Check sheet for the modelled part. Datum: model origin and axes. Units: mm. A direction names the side the tool comes from. Coordinates: 2 decimals unless noted, no trailing zeros. Order: outer loops, then holes, each group sorted by start corner. A loop starts at its lowest first (then second) coordinate and runs counter-clockwise, first axis right, second up.
1. Cross-section at C-C (y = -163.5). Enter the section's corners in (x, z), then the cut area to 3 significant figures.
2. Cross-section at D-D (y = -271). Enter the section's corners in (x, z).
3. Set-up check for faces 1 (the flat face through (2, -335, -29)), 2 (the flat face through (0, -165, 28)): record each of +Z, -Z, +X, -X, +Y, -Y from which the full face is reachable in a straight line by a thin tool's end or side.
4. Draft check along X on faces 3 (the flat face through (30, -165, 20)), 4 (the flat face through (28, -165, -19)), 5 (the flat face through (0, -165, -30)). Enter one of: released by +X, released by -X, zero draft, split by the parting line, or undercut.
5. Cross-section at B-B (x = 9). Enter the section's corners in (y, z), then the cut area to 3 significant figures.
6. Thickness scan on line 1 (Z direction, x = -20.5, y = -242.5). Record the ranges inside material, lowest first.
7. Cross-section at A-A (z = 9). Count the separate pieces of the cut face and the enclosed holes in it, then the cut area to 3 significant figures.
Autodesk Inventor part; units mm, degrees
ref_plane "YZ Plane" through (0, 0, 0) normal (1, 0, 0) x (0, 1, 0)
ref_plane "XZ Plane" through (0, 0, 0) normal (0, 1, 0) x (-1, 0, 0)
ref_plane "XY Plane" through (0, 0, 0) normal (0, 0, 1) x (1, 0, 0)
sketch "Sketch9" plane through (0, 0, 0) normal (0, 1, 0) x (-1, 0, 0)
  line L0 (30, 30) -> (-30, 30)
  line L1 (-30, 30) -> (-30, -30)
  line L2 (-30, -30) -> (30, -30)
  line L3 (30, -30) -> (30, 30)
  line L4 (30, 30) -> (-30, -30) construction
  line L5 (-30, 30) -> (30, -30) construction
  line L6 (-28, 28) -> (28, 28)
  line L7 (28, 28) -> (28, -28)
  line L8 (28, -28) -> (-28, -28)
  line L9 (-28, -28) -> (-28, 28)
  point P0 (0, 0)
  dimension "d172" = 60
  dimension "d173" = 60
  dimension "d174" = 2
extrude "Extrusion3" add sketch "Sketch9" against normal blind 335
sketch "Sketch10" plane through (0, 0, 0) normal (1, 0, 0) x (0, 1, 0)
  line L0 (0, 30) -> (0, -30) construction
  line L1 (0, 30) -> (-335, 30) construction
  line L2 (-335, -30) -> (-335, 30) construction
  line L3 (0, -30) -> (-335, -30) construction
  line L4 (-58.25, 15.25) -> (-27.75, 15.25)
  line L5 (-27.75, 15.25) -> (-27.75, -15.25)
  line L6 (-27.75, -15.25) -> (-58.25, -15.25)
  line L7 (-58.25, -15.25) -> (-58.25, 15.25)
  line L8 (-58.25, 15.25) -> (-27.75, -15.25) construction
  line L9 (-27.75, 15.25) -> (-58.25, -15.25) construction
  line L10 (-178.25, 15.25) -> (-147.75, 15.25)
  line L11 (-147.75, 15.25) -> (-147.75, -15.25)
  line L12 (-147.75, -15.25) -> (-178.25, -15.25)
  line L13 (-178.25, -15.25) -> (-178.25, 15.25)
  line L14 (-178.25, 15.25) -> (-147.75, -15.25) construction
  line L15 (-147.75, 15.25) -> (-178.25, -15.25) construction
  line L16 (-308.25, 15.25) -> (-277.75, 15.25)
  line L17 (-277.75, 15.25) -> (-277.75, -15.25)
  line L18 (-277.75, -15.25) -> (-308.25, -15.25)
  line L19 (-308.25, -15.25) -> (-308.25, 15.25)
  line L20 (-308.25, 15.25) -> (-277.75, -15.25) construction
  line L21 (-277.75, 15.25) -> (-308.25, -15.25) construction
  circle A0 centre (-453, 0) radius 9
  line L22 (0, 0) -> (47, 0)
  point P0 (-43, 0)
  point P1 (-163, 0)
  point P2 (-293, 0)
  dimension "d177" = 30.5
  dimension "d178" = 30.5
  dimension "d181" = 47
  dimension "d182" = 90
  dimension "d183" = 210
  dimension "d184" = 340
  dimension "d185" = 500
  dimension "d186" = 18
extrude "Extrusion4" cut sketch "Sketch10" along normal through all both and the other way through all contours L4 L5 L6 L7 | L10 L11 L12 L13 | L16 L17 L18 L19
sketch "Sketch11" plane through (30, 0, 30) normal (1, 0, 0) x (0, 0, -1)
  line L0 (45.25, -178.25) -> (14.75, -178.25)
  line L1 (14.75, -178.25) -> (14.75, -147.75)
  line L2 (14.75, -147.75) -> (45.25, -147.75)
  line L3 (45.25, -147.75) -> (45.25, -178.25)
  line L4 (45.25, -58.25) -> (14.75, -58.25)
  line L5 (14.75, -58.25) -> (14.75, -27.75)
  line L6 (14.75, -27.75) -> (45.25, -27.75)
  line L7 (45.25, -27.75) -> (45.25, -58.25)
  line L8 (45.25, -308.25) -> (14.75, -308.25)
  line L9 (14.75, -308.25) -> (14.75, -277.75)
  line L10 (14.75, -277.75) -> (45.25, -277.75)
  line L11 (45.25, -277.75) -> (45.25, -308.25)
  line L12 (0, 0) -> (60, 0)
  line L13 (0, 0) -> (0, -335)
  line L14 (60, -335) -> (0, -335)
  line L15 (60, 0) -> (60, -335)
  line L16 (45.25, -27.75) -> (14.75, -58.25)
  line L17 (45.25, -147.75) -> (14.75, -178.25)
  line L18 (45.25, -277.75) -> (14.75, -308.25)
  point P0 (30, 0)
sketch "Sketch13" plane through (-30, 0, -30) normal (-1, 0, 0) x (0, 0, 1)
  line L0 (45.25, -178.25) -> (14.75, -178.25)
  line L1 (14.75, -178.25) -> (14.75, -147.75)
  line L2 (14.75, -147.75) -> (45.25, -147.75)
  line L3 (45.25, -147.75) -> (45.25, -178.25)
  line L4 (45.25, -58.25) -> (14.75, -58.25)
  line L5 (14.75, -58.25) -> (14.75, -27.75)
  line L6 (14.75, -27.75) -> (45.25, -27.75)
  line L7 (45.25, -27.75) -> (45.25, -58.25)
  line L8 (45.25, -308.25) -> (14.75, -308.25)
  line L9 (14.75, -308.25) -> (14.75, -277.75)
  line L10 (14.75, -277.75) -> (45.25, -277.75)
  line L11 (45.25, -277.75) -> (45.25, -308.25)
  line L12 (0, 0) -> (60, 0)
  line L13 (0, 0) -> (0, -335)
  line L14 (60, -335) -> (0, -335)
  line L15 (60, 0) -> (60, -335)
  line L16 (14.75, -58.25) -> (45.25, -27.75)
  line L17 (14.75, -178.25) -> (45.25, -147.75)
  line L18 (14.75, -308.25) -> (45.25, -277.75)
  point P0 (30, 0)
fillet "Fillet1" radius 2 24 edges at (29, -277.75, -15.25) (29, -277.75, 15.25) (29, -308.25, 15.25) (29, -308.25, -15.25) (29, -178.25, -15.25) (29, -178.25, 15.25) (29, -147.75, 15.25) (29, -147.75, -15.25) (29, -58.25, 15.25) (29, -27.75, 15.25) (29, -27.75, -15.25) (29, -58.25, -15.25) (-29, -58.25, 15.25) (-29, -27.75, 15.25) (-29, -27.75, -15.25) (-29, -58.25, -15.25) (-29, -147.75, 15.25) (-29, -178.25, 15.25) (-29, -178.25, -15.25) (-29, -147.75, -15.25) (-29, -277.75, 15.25) (-29, -308.25, 15.25) (-29, -277.75, -15.25) (-29, -308.25, -15.25)
properties part number "TZS 1653 FDS 940 Diameter beam" material "Stainless Steel"
Data:
1. outline: (-30, -30) - (30, -30) - (30, -15.25) - (28, -15.25) - (28, -28) - (-28, -28) - (-28, -15.25) - (-30, -15.25) - close; (-30, 15.25) - (-28, 15.25) - (-28, 28) - (28, 28) - (28, 15.25) - (30, 15.25) - (30, 30) - (-30, 30) - close
1. area: 342 mm2
2. outline: (-30, -30) - (30, -30) - (30, 30) - (-30, 30) - close; hole (-28, -28) - (28, -28) - (28, 28) - (-28, 28) - close
3. face 1: +Z, -Z, +X, -X, -Y
3. face 2: +Y, -Y
4. face 3: released by +X
4. face 4: undercut
4. face 5: zero draft
5. outline: (-335, -30) - (0, -30) - (0, -28) - (-335, -28) - close; (-335, 28) - (0, 28) - (0, 30) - (-335, 30) - close
5. area: 1,340 mm2
6. line 1: z = -30 to -28, 28 to 30
7. separate pieces: 8
7. enclosed holes: 0
7. area: 974 mm2
